```python
from build123d import *

# Parameters (mm, degrees)
SKETCH1_W           = 479
SKETCH1_H           = 721
SKETCH1_W_2         = 419
SKETCH1_H_2         = 419
SKETCH1_W_3         = 196
SKETCH1_H_3         = 112
BOSS_EXTRUDE1_DEPTH = 3.175
CUT_EXTRUDE1_DEPTH  = 441.375774197
SKETCH3_R           = 1.375
CUT_EXTRUDE2_DEPTH  = 441.375774197


with BuildPart() as part:
    # Sketch1 → Boss-Extrude1 (new, symmetric)
    with BuildSketch(Plane(origin=(0, 0, 0), x_dir=(1, 0, 0), z_dir=(0, 1, 0))):
        with Locations((0, 9)):
            Rectangle(SKETCH1_W, SKETCH1_H)
        Rectangle(SKETCH1_W_2, SKETCH1_H_2, mode=Mode.SUBTRACT)
        with Locations((0, -285.5)):
            Rectangle(SKETCH1_W_3, SKETCH1_H_3, mode=Mode.SUBTRACT)
    extrude(amount=BOSS_EXTRUDE1_DEPTH, both=True)

    # Sketch2 → Cut-Extrude1 (cut, through all)
    with BuildSketch(Plane(origin=(0, 3.175, 0), x_dir=(1, 0, 0), z_dir=(0, 1, 0))):
        Polygon((-239.5, 369.5), (-239.5, 269.5), (-233.15, 269.5), (-233.15, 363.15), (-139.5, 363.15), (-139.5, 369.5), align=None)
        Polygon((239.5, 369.5), (139.5, 369.5), (139.5, 363.15), (233.15, 363.15), (233.15, 269.5), (239.5, 269.5), align=None)
        Polygon((239.5, -351.5), (239.5, -251.5), (233.15, -251.5), (233.15, -345.15), (139.5, -345.15), (139.5, -351.5), align=None)
        Polygon((-239.5, -351.5), (-139.5, -351.5), (-139.5, -345.15), (-233.15, -345.15), (-233.15, -251.5), (-239.5, -251.5), align=None)
    extrude(amount=-CUT_EXTRUDE1_DEPTH, mode=Mode.SUBTRACT)

    # Sketch3 → Cut-Extrude2 (cut, through all)
    with BuildSketch(Plane(origin=(0, 3.175, 0), x_dir=(1, 0, 0), z_dir=(0, 1, 0))):
        with Locations(Location((166.32, 240.12, 0), (0, 0, 270))):
            Circle(SKETCH3_R)
        with Locations(Location((201.88, 240.12, 0), (0, 0, 270))):
            Circle(SKETCH3_R)
    extrude(amount=-CUT_EXTRUDE2_DEPTH, mode=Mode.SUBTRACT)


solid = part.part
```
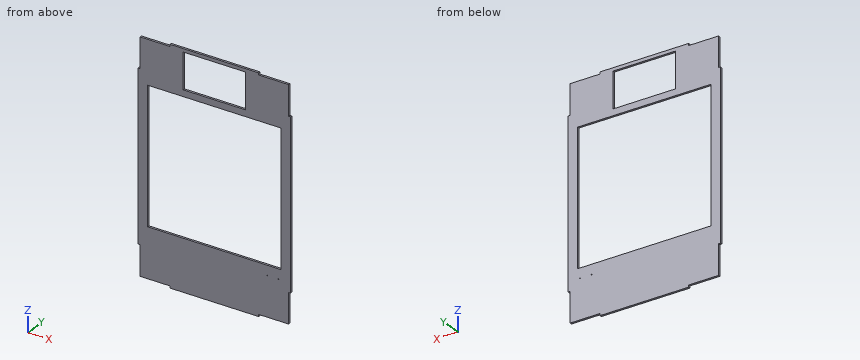
For this review, take the finished solid that the model builds, in its own axes (mm). Round coordinates to 2 decimals unless told otherwise and drop trailing zeros. Loops run counter-clockwise (first coordinate to the right, second up) from the corner with the lowest first, then second, coordinate; pieces in that order, holes last.
Q1. Insertion check: pin 1 Ø3 at (x, y) = (202.5, -1.5) entering from -Z; pin 2 Ø1.9 at (y, z) = (0, -366.5) entering from +X; pin 3 Ø3 at (x, y) = (208.5, 1) entering from +Z; pin 4 Ø2.5 at (x, z) = (166.32, -240.12) entering from +Y. Each pin has a flat end and moves straight along its axis. Give the tip position at first contact, or say it passes through.
Result sheet:
pin 1: stops at z = -363.15
pin 2: stops at x = 139.5
pin 3: stops at z = 345.15
pin 4: passes through
Q2. Add section D-D on x = -73. Write out the cut boundary in (y, z) (3 decimals), plus the area to 3 significant figures.
Result sheet:
outline: (-3.175, -369.5) - (3.175, -369.5) - (3.175, -209.5) - (-3.175, -209.5) - close; (-3.175, 209.5) - (3.175, 209.5) - (3.175, 229.5) - (-3.175, 229.5) - close; (-3.175, 341.5) - (3.175, 341.5) - (3.175, 351.5) - (-3.175, 351.5) - close
area: 1,210 mm2
Q3. Add section A-A on z = -46. Write out the cut boundary in (x, y) (3 decimals), plus the area to 3 significant figures.
Result sheet:
outline: (-239.5, -3.175) - (-209.5, -3.175) - (-209.5, 3.175) - (-239.5, 3.175) - close; (209.5, -3.175) - (239.5, -3.175) - (239.5, 3.175) - (209.5, 3.175) - close
area: 381 mm2
Q4. Add section C-C on y = -1.5. Give the number of separate pieces and of enclosed holes in the cut face, plus the area to 3 significant figures.
Result sheet:
separate pieces: 1
enclosed holes: 4
area: 143,000 mm2
Q5. Add section B-B on x = 184. Write out the cut boundary in (y, z) (3 decimals).
Result sheet:
outline: (-3.175, -363.15) - (3.175, -363.15) - (3.175, -209.5) - (-3.175, -209.5) - close; (-3.175, 209.5) - (3.175, 209.5) - (3.175, 345.15) - (-3.175, 345.15) - close
Q6. To check wall thickness, follow line 1 along Z through (x, y) = (201.88, -0.25) (3 decimals); line 2 along Z through (x, y) = (70, 1.75); line 3 along X through (y, z) = (-1.25, -240.12) (3 decimals). State the ranges of each line that lie inside material, in increasing order.
Result sheet:
line 1: z = -363.15 to -241.495, -238.745 to -209.5, 209.5 to 345.15
line 2: z = -369.5 to -209.5, 209.5 to 229.5, 341.5 to 351.5
line 3: x = -239.5 to 164.945, 167.695 to 200.505, 203.255 to 239.5
